The model under review builds one solid part; all positions refer to its coordinate system, in mm. Face numbers are marked on the shaded views. A direction names the side the tool comes from. Give positions to 0.01 mm unless a question says otherwise; leave off trailing zeros. Order: outer loops, then holes, each group sorted by start corner. A loop starts at its lowest first (then second) coordinate and runs counter-clockwise, first axis right, second up. Notation, with made-up numbers: M 78,72.25 L 107,72.25 A21 ccw 107,104.25 Z; hole C -19,49 d7. An arc over 180 degrees is marked long. One line per question, with ' | ' between items. Start each with the question number.
1. Insertion check: P1, Ø3, axis at y = 28, z = -8.5, coming from the +X side; P2, Ø3.5, axis at y = -2, z = 5.5, coming from the +X side; P3, Ø5, axis at x = -8, z = -2.5, coming from the +Y side; P4, Ø7.5, axis at x = 2, z = 0, coming from the -Y side. Each pin has a flat end and moves straight along its axis. Give the tip position at first contact, or say it passes through.
2. The part is to be moulded in two halves that separate along X. For the marked faces 1, 2, 3 and 4, say which applies: +X half, -X half, draft (parallel to the pull), parting line (faces both ways), or undercut.
3. Wall thickness on L1, parallel to Z at x = 2, y = -1; L2, parallel to X at y = 3, z = 0; L3, parallel to Y at x = 7.5, z = 11: over which ranges is each line inside the solid? List them lowest first.
4. For the marked faces 5, 6 and 7, list the 3-axis set-ups (+Z, -Z, +X, -X, +Y, -Y) from which the entire face can be reached by the end or side of a thin tool; tool diameter is ignored.
5. We need section C-C on z = -5.5. Write out the cut boundary in (x, y), then the cut area to 3 significant figures.
6. We need section A-A on x = 2. Write out the cut boundary in (y, z).
7. We need section D-D on x = 18.5. Write out the cut boundary in (y, z).
8. We need section B-B on z = 0. Write out the cut boundary in (x, y), then the cut area to 3 significant figures.
Autodesk Inventor part; units mm, degrees
ref_plane "YZ Plane" through (0, 0, 0) normal (1, 0, 0) x (0, 1, 0)
ref_plane "XZ Plane" through (0, 0, 0) normal (0, 1, 0) x (-1, 0, 0)
ref_plane "XY Plane" through (0, 0, 0) normal (0, 0, 1) x (1, 0, 0)
sketch "Sketch1" plane through (0, 0, 0) normal (0, 1, 0) x (-1, 0, 0)
  line L0 (-22, 20) -> (22, 20)
  line L1 (22, 20) -> (22, -20)
  line L2 (22, -20) -> (-22, -20)
  line L3 (-22, -20) -> (-22, 20)
  line L4 (-22, 20) -> (22, -20) construction
  line L5 (22, 20) -> (-22, -20) construction
  point P0 (0, 0)
  dimension "d0" = 44
  dimension "d1" = 40
extrude "Extrusion1" add sketch "Sketch1" along normal blind 5
sketch "Sketch2" plane through (0, 0, 0) normal (0, -1, 0) x (1, 0, 0)
  line L0 (22, -20) -> (-22, -20)
  line L1 (-22, 20) -> (22, 20)
  line L2 (-3, -20) -> (7, -20)
  line L3 (7, -20) -> (7, 20)
  line L4 (7, 20) -> (-3, 20)
  line L5 (-3, 20) -> (-3, -20)
  line L6 (22, 20) -> (22, -20)
  point P0 (-3, 20)
  dimension "d7" = 10
  dimension "d8" = 15
extrude "Extrusion2" add sketch "Sketch2" along normal blind 3 contours L0 L5 L1 L3
sketch "Sketch3" plane through (0, 5, 0) normal (0, 1, 0) x (1, 0, 0)
  line L0 (-22, -20) -> (22, -20)
  line L1 (-22, -20) -> (-17, -20)
  line L2 (-17, -20) -> (-17, 20)
  line L3 (-17, 20) -> (-22, 20)
  line L4 (-22, 20) -> (-22, -20)
  point P0 (0, 0)
  point P1 (-17, -20)
  dimension "d9" = 5
  dimension "d10" = 40
extrude "Extrusion3" add sketch "Sketch3" along normal blind 30
sketch "Sketch4" plane through (0, 5, 0) normal (0, 1, 0) x (1, 0, 0)
  line L0 (22, -20) -> (22, 20)
  point P0 (0, 0)
  point P1 (2, 0)
  point P2 (22, 0)
  dimension "d13" = 20
hole "Hole1" at (2, 5, 0) direction (0, -1, 0) diameter 8.6 end through all
properties part number "ER_Stopper_Rexroth"
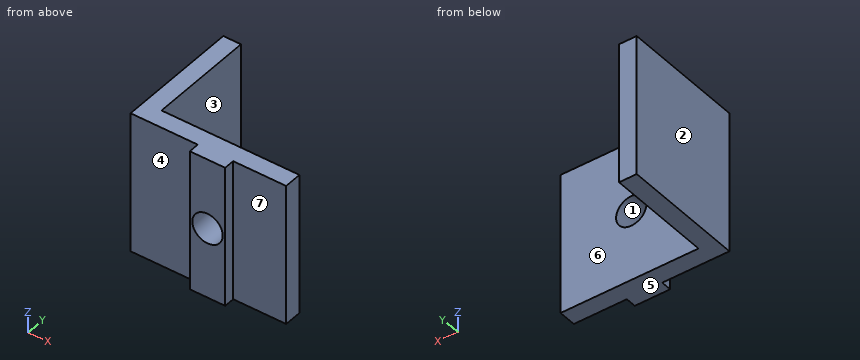
Entries:
1) P1: stops at x = -17 | P2: stops at x = 7 | P3: stops at y = 5 | P4: passes through
2) face 1: undercut | face 2: -X half | face 3: +X half | face 4: draft
3) L1: z = -20 to -4.3, 4.3 to 20 | L2: x = -22 to -2.3, 6.3 to 22 | L3: y = 0 to 5
4) face 5: -Z, +X, -X, +Y, -Y | face 6: +Z, -Z, +X, +Y | face 7: +Z, -Z, +X, -Y
5) outline: M -22,0 L -3,0 L -3,-3 L 7,-3 L 7,0 L 22,0 L 22,5 L -17,5 L -17,35 L -22,35 Z | area: 400 mm^2
6) outline: M -3,-20 L 5,-20 L 5,-4.3 L -3,-4.3 Z; M -3,4.3 L 5,4.3 L 5,20 L -3,20 Z
7) outline: M 0,-20 L 5,-20 L 5,20 L 0,20 Z
8) outline: M -22,0 L -3,0 L -3,-3 L -2.3,-3 L -2.3,5 L -17,5 L -17,35 L -22,35 Z; M 6.3,-3 L 7,-3 L 7,0 L 22,0 L 22,5 L 6.3,5 Z | area: 331 mm^2
